Here's how the part is built. I have some questions about the finished solid (model axes, mm). A direction names the side the tool comes from. Round coordinates to 2 decimals unless told otherwise and drop trailing zeros. Write each loop counter-clockwise with the first axis right and the second up, starting at its lowest first coordinate (ties: lowest second). Pieces come first, ordered by that corner, then holes. Notation, with made-up numbers: (-2.5, 5.5) - (28.5, 5.5) arc R30 cw to (28.5, 33.5) - close; hole circle Ø9 at (75.25, -18). An arc over 180 degrees is marked (long way). Use one line per item in the form item = value. Start each with the question number.
1. Will these pins go through, and if not, where does the flat tip stop? pin 1 (1.5 mm diameter, centred on y = 6, z = 9, fed in from +X); pin 2 (1 mm diameter, centred on x = 70, y = 18, fed in from +Z).
2. If I drill on line 1 along Y through (x, z) = (18.5, 12); line 2 along X through (y, z) = (18.5, 4.75), over which ranges is the centre line in solid material (lowest first)?
3. We'd pull the mould along Y, two halves only. Please class faces 1 (the flat face through (41, 26, 9)), 2 (the flat face through (3, 13, 10)), 3 (the flat face through (83, 13, 1)): +Y half, -Y half, draft (parallel to the pull), parting line (faces both ways), or undercut.
4. I want a section at A-A, the plane x = 26.5. List the corners of the cut face in (y, z) for me, plus the area to 3 significant figures.
5. Which directions (+Z, -Z, +X, -X, +Y, -Y) give clear straight access to the entire face, cutting with the end or side of a thin tool? Please do faces 4 (the flat face through (42, 13, 3)), 5 (the flat face through (35, 2, 18)).
6. I want a section at B-B, the plane z = 15.75. List the corners of the cut face in (x, y) for me, plus the area to 3 significant figures.
7. I want a section at C-C, the plane y = 18.5. List the corners of the cut face in (x, z) for me.
```python
from build123d import *

# Parameters (mm, degrees)
BOX003_W     = 3
BOX003_H     = 26
BOX003_DEPTH = 18
BOX_W        = 83
BOX_H        = 26
BOX_DEPTH    = 3
BOX001_W     = 83
BOX001_H     = 3
BOX001_DEPTH = 18
BOX002_W     = 83
BOX002_H     = 3
BOX002_DEPTH = 18


with BuildPart() as obj1:
    # Box003 → Box003 (new body)
    with BuildSketch(Plane.XY):
        with Locations((1.5, 13)):
            Rectangle(BOX003_W, BOX003_H)
    extrude(amount=BOX003_DEPTH)


with BuildPart() as baseinferior:
    # Box → Box (new body)
    with BuildSketch(Plane.XY):
        with Locations((41.5, 13)):
            Rectangle(BOX_W, BOX_H)
    extrude(amount=BOX_DEPTH)


with BuildPart() as obj2:
    # Box001 → Box001 (new body)
    with BuildSketch(Plane.XY):
        with Locations((41.5, 1.5)):
            Rectangle(BOX001_W, BOX001_H)
    extrude(amount=BOX001_DEPTH)


with BuildPart() as obj3:
    # Box002 → Box002 (new body)
    with BuildSketch(Plane(origin=(0, 23, 0), x_dir=(1, 0, 0), z_dir=(0, 0, 1))):
        with Locations((41.5, 1.5)):
            Rectangle(BOX002_W, BOX002_H)
    extrude(amount=BOX002_DEPTH)

    # Fusion: union obj1, BaseInferior, obj2
    add(obj1.part)
    add(baseinferior.part)
    add(obj2.part)


solid = obj3.part
```
Model answer:
q1.pin_1 = 3
q1.pin_2 = 3
q2.line_1 = 0 to 3, 23 to 26
q2.line_2 = 0 to 3
q3.face_1 = +Y half
q3.face_2 = undercut
q3.face_3 = draft
q4.outline = (0, 0) - (26, 0) - (26, 18) - (23, 18) - (23, 3) - (3, 3) - (3, 18) - (0, 18) - close
q4.area = 168 mm2
q5.face_4 = +Z, +X
q5.face_5 = +Z, +X, -X, +Y, -Y
q6.outline = (0, 0) - (83, 0) - (83, 3) - (3, 3) - (3, 23) - (83, 23) - (83, 26) - (0, 26) - close
q6.area = 558 mm2
q7.outline = (0, 0) - (83, 0) - (83, 3) - (3, 3) - (3, 18) - (0, 18) - close
